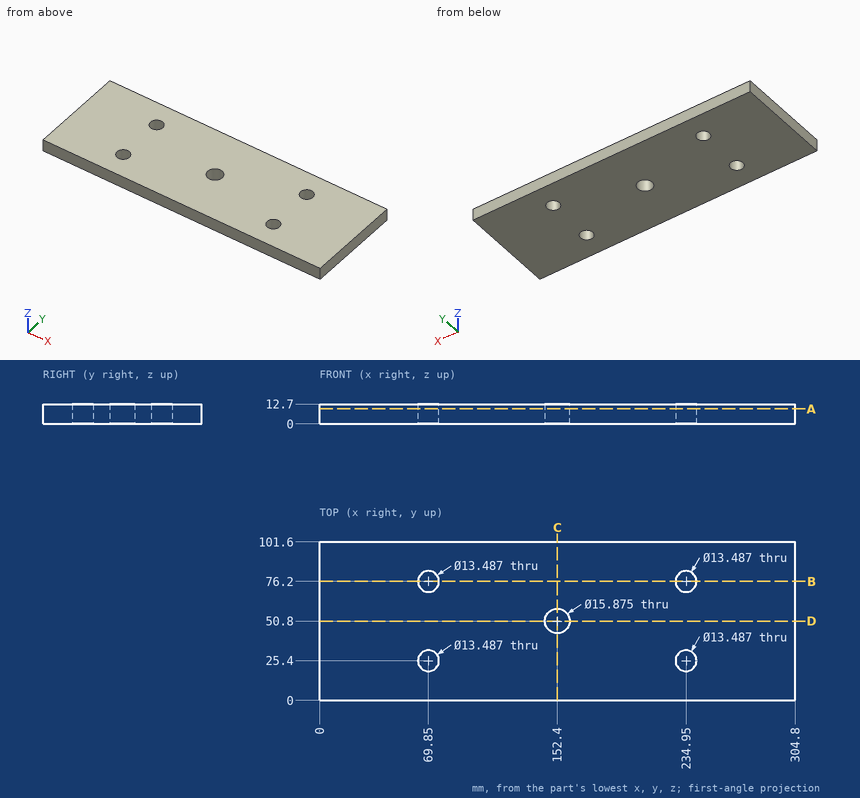
Study the drawing (mm; zero at the part's minimum x, y, z) and answer. Coordinates: 2 decimals unless noted, no trailing zeros. Loops run counter-clockwise (first coordinate to the right, second up) from the corner with the lowest first, then second, coordinate; pieces in that order, holes last. Notation, with made-up numbers: (60, 88) -> (72, 88) arc R32 ccw to (72, 115) -> close; hole circle Ø7 at (2.5, 76). An arc over 180 degrees is marked (long way). Write item = value, one per line. Start each with the question number.
1) Find the intervals of material crossed by L1, parallel to Y at x = 69.85, z = 9.75; L2, parallel to X at y = 81, z = 8.5 (1 decimal); L3, parallel to X at y = 74.5, z = 6.5 (1 decimal), in increasing order. Write a range as from..to.
2) The part is cut by section C-C, the plane x = 152.4. Determine the outline of the cut face in (y, z), plus the area to 3 significant figures.
3) The part is cut by section A-A, the plane z = 9.5. State how many separate pieces and enclosed holes the cut face has, plus the area to 3 significant figures.
4) The part is cut by section B-B, the plane y = 76.2. Determine the outline of the cut face in (x, z).
5) The part is cut by section D-D, the plane y = 50.8. Determine the outline of the cut face in (x, z).
Result:
q1.L1 = 0..18.66, 32.14..69.46, 82.94..101.6
q1.L2 = 0..65.1, 74.6..230.2, 239.7..304.8
q1.L3 = 0..63.3, 76.4..228.4, 241.5..304.8
q2.outline = (0, 0) -> (42.86, 0) -> (42.86, 12.7) -> (0, 12.7) -> close; (58.74, 0) -> (101.6, 0) -> (101.6, 12.7) -> (58.74, 12.7) -> close
q2.area = 1,090 mm²
q3.separate_pieces = 1
q3.enclosed_holes = 5
q3.area = 30,200 mm²
q4.outline = (0, 0) -> (63.11, 0) -> (63.11, 12.7) -> (0, 12.7) -> close; (76.59, 0) -> (228.21, 0) -> (228.21, 12.7) -> (76.59, 12.7) -> close; (241.69, 0) -> (304.8, 0) -> (304.8, 12.7) -> (241.69, 12.7) -> close
q5.outline = (0, 0) -> (144.46, 0) -> (144.46, 12.7) -> (0, 12.7) -> close; (160.34, 0) -> (304.8, 0) -> (304.8, 12.7) -> (160.34, 12.7) -> close
